Build history of the part. All positions in model axes, mm. Round coordinates to 2 decimals unless told otherwise and drop trailing zeros. Write each loop counter-clockwise with the first axis right and the second up, starting at its lowest first coordinate (ties: lowest second). Pieces come first, ordered by that corner, then holes.
Item 1: Wall check: probe 1 along X at (y, z) = (154, 1.5); probe 2 along X at (y, z) = (105.5, 5.5); probe 3 along Y at (x, z) = (17.7, 4.5). Give the ranges that are in metal, low to high.
Item 2: Drop flat-ended pins along their axis: pin 1 Ø1.6 at (x, z) = (102, 2.5) entering from -Y; pin 2 Ø0.9 at (x, z) = (-5.5, 4) entering from -Y; pin 3 Ø1 at (y, z) = (142.5, 4) entering from +X; pin 4 Ø4.5 at (x, y) = (17.7, 124.96) entering from -Z. Give the stop position or say it passes through.
Item 3: Band-saw the part on A-A, the plane y = 208. Write the cut outline in (x, z).
Item 4: Band-saw the part on C-C, the plane y = 147. Write the cut outline in (x, z), then the cut area to 3 significant figures.
Item 5: Band-saw the part on B-B, the plane x = 17.7. Write the cut outline in (y, z).
Item 6: Band-saw the part on D-D, the plane z = 1.5. Count the separate pieces of the cut face and the enclosed holes in it, then the cut area to 3 significant figures.
Autodesk Inventor part; units mm, degrees
ref_plane "YZ Plane" through (0, 0, 0) normal (1, 0, 0) x (0, 1, 0)
ref_plane "XZ Plane" through (0, 0, 0) normal (0, 1, 0) x (-1, 0, 0)
ref_plane "XY Plane" through (0, 0, 0) normal (0, 0, 1) x (1, 0, 0)
sketch "Sketch1" plane through (0, 0, 0) normal (0, 0, 1) x (1, 0, 0)
  line L0 (0, 0) -> (95.25, 0)
  line L1 (95.25, 0) -> (95.25, 198.2931)
  line L2 (95.25, 198.2931) -> (0, 198.2931)
  line L3 (0, 198.2931) -> (0, 0)
  line L4 (0, 198.2931) -> (95.25, 253.2857)
  line L5 (95.25, 253.2857) -> (95.25, 198.2646)
  dimension "d0" = 95.25
  dimension "d1" = 198.293
  dimension "d2" = 60
extrude "Extrusion1" add sketch "Sketch1" along normal blind 6.35
sketch "Sketch2" plane through (0, 0, 6.35) normal (0, 0, 1) x (1, 0, 0)
  line L0 (0, 198.2931) -> (0, 0)
  line L1 (0, 38.1146) -> (-7.62, 38.1146)
  line L2 (-7.62, 38.1146) -> (-7.62, 12.7146)
  line L3 (-7.62, 12.7146) -> (0, 12.7146)
  line L4 (0, 12.7146) -> (0, 38.1146)
  line L5 (0, 165.1146) -> (-7.62, 165.1146)
  line L6 (-7.62, 165.1146) -> (-7.62, 139.7146)
  line L7 (-7.62, 139.7146) -> (0, 139.7146)
  line L8 (0, 139.7146) -> (0, 165.1146)
  line L9 (0, 0) -> (95.25, 0)
  dimension "d5" = 7.62
  dimension "d6" = 25.4
  dimension "d7" = 25.4
  dimension "d8" = 101.6
  dimension "d9" = 12.7146
extrude "Extrusion2" add sketch "Sketch2" against normal blind 6.35
sketch "Sketch3" plane through (0, 0, 6.35) normal (0, 0, 1) x (1, 0, 0)
  line L0 (95.25, 0) -> (95.25, 253.2857)
  line L1 (95.25, 228.6) -> (102.87, 228.6)
  line L2 (102.87, 228.6) -> (102.87, 203.2)
  line L3 (102.87, 203.2) -> (95.25, 203.2)
  line L4 (95.25, 203.2) -> (95.25, 228.6)
  line L5 (95.25, 50.8) -> (102.87, 50.8)
  line L6 (102.87, 50.8) -> (102.87, 25.4)
  line L7 (102.87, 25.4) -> (95.25, 25.4)
  line L8 (95.25, 25.4) -> (95.25, 50.8)
  line L9 (102.87, 215.9) -> (102.87, 38.1) construction
  line L10 (0, 0) -> (95.25, 0)
  point P0 (102.87, 127)
  point P1 (95.25, 126.6428)
  dimension "d13" = 25.4
  dimension "d14" = 7.62
  dimension "d15" = 25.4
  dimension "d16" = 177.8
  dimension "d19" = 25.4
extrude "Extrusion3" add sketch "Sketch3" against normal blind 6.35
sketch "Sketch4" plane through (0, 0, 6.35) normal (0, 0, 1) x (1, 0, 0)
  circle A0 centre (17.7, 124.9622) radius 2.5
  circle A1 centre (17.7, 57.4622) radius 2.5
  line L0 (0, 139.7146) -> (0, 38.1146)
  line L1 (0, 0) -> (95.25, 0)
  dimension "d20" = 5
  dimension "d21" = 5
  dimension "d22" = 17.7
  dimension "d23" = 67.5
  dimension "d24" = 57.4622
extrude "Extrusion4" cut sketch "Sketch4" against normal through all
sketch "Sketch5" plane through (0, 0, 6.35) normal (0, 0, 1) x (1, 0, 0)
  circle A0 centre (47.625, 198.2931) radius 12.5
  line L0 (0, 0) -> (95.25, 0)
  point P0 (0, 198.2931)
  point P1 (47.625, 0)
  dimension "d27" = 25
extrude "Extrusion5" cut sketch "Sketch5" against normal through all
sketch "Sketch6" plane through (0, 0, 6.35) normal (0, 0, 1) x (1, 0, 0)
  circle A0 centre (47.625, 198.2931) radius 12.5 construction
  circle A1 centre (17.7, 124.9622) radius 2.5 construction
  circle A2 centre (17.7, 57.4622) radius 2.5 construction
  line L0 (95.25, 0) -> (95.25, 25.4) construction
  line L1 (95.25, 25.4) -> (102.87, 25.4) construction
  line L2 (102.87, 25.4) -> (102.87, 50.8) construction
  line L3 (102.87, 50.8) -> (95.25, 50.8) construction
  line L4 (95.25, 50.8) -> (95.25, 203.2) construction
  line L5 (95.25, 203.2) -> (102.87, 203.2) construction
  line L6 (102.87, 203.2) -> (102.87, 228.6) construction
  line L7 (102.87, 228.6) -> (95.25, 228.6) construction
  line L8 (95.25, 228.6) -> (95.25, 253.2857) construction
  line L9 (95.25, 253.2857) -> (0, 198.2931) construction
  line L10 (0, 198.2931) -> (0, 165.1146) construction
  line L11 (0, 165.1146) -> (-7.62, 165.1146) construction
  line L12 (-7.62, 165.1146) -> (-7.62, 139.7146) construction
  line L13 (-7.62, 139.7146) -> (0, 139.7146) construction
  line L14 (0, 139.7146) -> (0, 38.1146) construction
  line L15 (0, 38.1146) -> (-7.62, 38.1146) construction
  line L16 (-7.62, 38.1146) -> (-7.62, 12.7146) construction
  line L17 (-7.62, 12.7146) -> (0, 12.7146) construction
  line L18 (0, 12.7146) -> (0, 0) construction
  line L19 (0, 0) -> (95.25, 0) construction
  line L20 (-2.2451, 167.3597) -> (-2.2451, 199.5892) construction
  line L21 (-2.2451, 199.5892) -> (97.4951, 257.1742) construction
  line L22 (97.4951, 257.1742) -> (97.4951, 230.8451) construction
  line L23 (97.4951, 230.8451) -> (105.1151, 230.8451) construction
  line L24 (105.1151, 230.8451) -> (105.1151, 200.9549) construction
  line L25 (105.1151, 200.9549) -> (97.4951, 200.9549) construction
  line L26 (97.4951, 200.9549) -> (97.4951, 53.0451) construction
  line L27 (97.4951, 53.0451) -> (105.1151, 53.0451) construction
  line L28 (105.1151, 53.0451) -> (105.1151, 23.1549) construction
  line L29 (105.1151, 23.1549) -> (97.4951, 23.1549) construction
  line L30 (97.4951, 23.1549) -> (97.4951, -2.2451) construction
  line L31 (97.4951, -2.2451) -> (-2.2451, -2.2451) construction
  line L32 (-2.2451, -2.2451) -> (-2.2451, 10.4695) construction
  line L33 (-2.2451, 10.4695) -> (-9.8651, 10.4695) construction
  line L34 (-9.8651, 10.4695) -> (-9.8651, 40.3597) construction
  line L35 (-9.8651, 40.3597) -> (-2.2451, 40.3597) construction
  line L36 (-2.2451, 40.3597) -> (-2.2451, 137.4695) construction
  line L37 (-2.2451, 137.4695) -> (-9.8651, 137.4695) construction
  line L38 (-9.8651, 137.4695) -> (-9.8651, 167.3597) construction
  line L39 (-9.8651, 167.3597) -> (-2.2451, 167.3597) construction
  circle A3 centre (97.4951, 230.8451) radius 3.175
  line L40 (95.25, 50.8) -> (95.25, 203.2)
  circle A4 centre (97.4951, 200.9549) radius 3.175
  circle A5 centre (97.4951, 53.0451) radius 3.175
  circle A6 centre (97.4951, 23.1549) radius 3.175
  line L41 (0, 12.7146) -> (0, 0)
  circle A7 centre (-2.2451, 10.4695) radius 3.175
  line L42 (0, 139.7146) -> (0, 38.1146)
  circle A8 centre (-2.2451, 40.3597) radius 3.175
  circle A9 centre (-2.2451, 137.4695) radius 3.175
  line L43 (0, 198.2931) -> (0, 165.1146)
  circle A10 centre (-2.2451, 167.3597) radius 3.175
  dimension "d30" = 6.35
extrude "Extrusion6" cut sketch "Sketch6" against normal through all
equation "\"d3\" = Panel_Thickness"
equation "\"d5\" = Panel_Thickness + Fit_Tolerance"
equation "\"d10\" = Panel_Thickness"
equation "\"d14\" = Panel_Thickness + Fit_Tolerance"
equation "\"d17\" = Panel_Thickness"
equation "\"d25\" = Panel_Thickness"
equation "\"d28\" = Panel_Thickness"
equation "\"d30\" = Tool_Dia"
equation "\"d31\" = Panel_Thickness"
equation "\"Panel_Thickness\" = 6.35"
equation "\"Fit_Tolerance\" = 1.27"
equation "\"Tool_Dia\" = 6.35"
properties part number "BA23" material "Polyethylene, High Density"
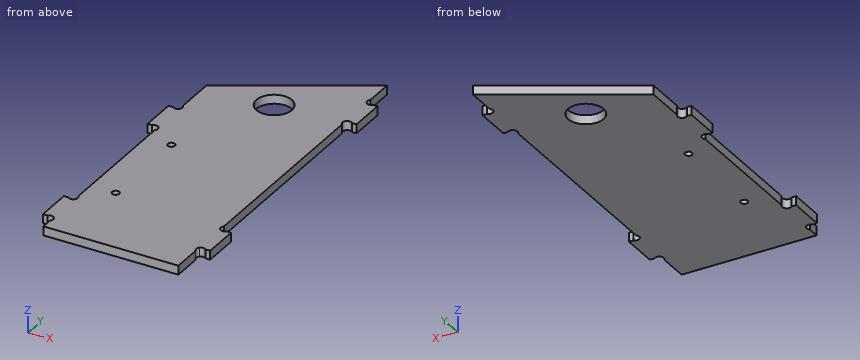
Results:
1. probe 1: x = -7.62 to 95.25
1. probe 2: x = 0 to 95.25
1. probe 3: y = 0 to 54.96, 59.96 to 122.46, 127.46 to 208.51
2. pin 1: stops at y = 25.4
2. pin 2: stops at y = 12.71
2. pin 3: stops at x = 95.25
2. pin 4: passes through
3. outline: (16.81, 0) - (39.75, 0) - (39.75, 6.35) - (16.81, 6.35) - close; (55.5, 0) - (102.87, 0) - (102.87, 6.35) - (55.5, 6.35) - close
4. outline: (-7.62, 0) - (95.25, 0) - (95.25, 6.35) - (-7.62, 6.35) - close
4. area: 653 mm2
5. outline: (0, 0) - (54.96, 0) - (54.96, 6.35) - (0, 6.35) - close; (59.96, 0) - (122.46, 0) - (122.46, 6.35) - (59.96, 6.35) - close; (127.46, 0) - (208.51, 0) - (208.51, 6.35) - (127.46, 6.35) - close
6. separate pieces: 1
6. enclosed holes: 3
6. area: 21,700 mm2
